```python
from build123d import *

# Parameters (mm, degrees)
BOSS_EXTRUDE1_DEPTH             = 3.175
F_6_CLEARANCE_HOLE1_AT_2_COUNT  = 2
F_6_CLEARANCE_HOLE1_AT_2_PITCH  = 202.184
F_6_CLEARANCE_HOLE1_AT_3_COUNT  = 2
F_6_CLEARANCE_HOLE1_AT_3_PITCH  = 245.533205315
F_6_CLEARANCE_HOLE1_AT_4_COUNT  = 2
F_6_CLEARANCE_HOLE1_AT_4_PITCH  = 294.732330958
F_6_CLEARANCE_HOLE1_AT_5_COUNT  = 2
F_6_CLEARANCE_HOLE1_AT_5_PITCH  = 209.296
F_6_CLEARANCE_HOLE1_AT_6_COUNT  = 2
F_6_CLEARANCE_HOLE1_AT_6_PITCH  = 172.811757411
F_6_CLEARANCE_HOLE1_AT_7_COUNT  = 2
F_6_CLEARANCE_HOLE1_AT_7_PITCH  = 57.300187604
F_6_CLEARANCE_HOLE1_AT_8_COUNT  = 2
F_6_CLEARANCE_HOLE1_AT_8_PITCH  = 291.003755082
F_6_CLEARANCE_HOLE1_AT_9_COUNT  = 2
F_6_CLEARANCE_HOLE1_AT_9_PITCH  = 232.431512666
F_6_CLEARANCE_HOLE1_AT_10_COUNT = 2
F_6_CLEARANCE_HOLE1_AT_10_PITCH = 101.092
SKETCH23_R                      = 24.765
CUT_EXTRUDE10_DEPTH             = 191.76187976
SKETCH24_W                      = 59.69
SKETCH24_H                      = 45.212
CUT_EXTRUDE11_DEPTH             = 191.76187976
FILLET2_R                       = 4.699
CHAMFER1_SIZE                   = 1.905
M3_CLEARANCE_HOLE3_AT_2_COUNT   = 2
M3_CLEARANCE_HOLE3_AT_2_PITCH   = 49.391408666
M3_CLEARANCE_HOLE3_AT_3_COUNT   = 2
M3_CLEARANCE_HOLE3_AT_3_PITCH   = 69.85
M3_CLEARANCE_HOLE3_AT_4_COUNT   = 2
M3_CLEARANCE_HOLE3_AT_4_PITCH   = 49.391408666
M3_CLEARANCE_HOLE1_D            = 3.6
M3_CLEARANCE_HOLE1_CSINK_D      = 5.7
M3_CLEARANCE_HOLE1_CSINK_ANGLE  = 90
M3_CLEARANCE_HOLE2_AT_2_COUNT   = 2
M3_CLEARANCE_HOLE2_AT_2_PITCH   = 56.70042
M3_CLEARANCE_HOLE2_AT_3_COUNT   = 2
M3_CLEARANCE_HOLE2_AT_3_PITCH   = 102.00589147
M3_CLEARANCE_HOLE2_AT_4_COUNT   = 2
M3_CLEARANCE_HOLE2_AT_4_PITCH   = 109.267844742
M3_CLEARANCE_HOLE2_AT_5_COUNT   = 2
M3_CLEARANCE_HOLE2_AT_5_PITCH   = 65.600653918
M3_CLEARANCE_HOLE2_AT_6_COUNT   = 2
M3_CLEARANCE_HOLE2_AT_6_PITCH   = 76.404880698
M3_CLEARANCE_HOLE2_AT_7_COUNT   = 2
M3_CLEARANCE_HOLE2_AT_7_PITCH   = 27.404059918
M3_CLEARANCE_HOLE2_AT_8_COUNT   = 2
M3_CLEARANCE_HOLE2_AT_8_PITCH   = 55.968061912
SKETCH35_W                      = 13.335
SKETCH35_H                      = 28.575
CUT_EXTRUDE12_DEPTH             = 191.76187976
FILLET1_R                       = 1.5875
F_8_0MM_DOWEL_HOLE1_D           = 8
M3_CLEARANCE_HOLE4_AT_2_COUNT   = 2
M3_CLEARANCE_HOLE4_AT_2_PITCH   = 78.105
M3_CLEARANCE_HOLE4_AT_3_COUNT   = 2
M3_CLEARANCE_HOLE4_AT_3_PITCH   = 97.157075141
M3_CLEARANCE_HOLE4_AT_4_COUNT   = 2
M3_CLEARANCE_HOLE4_AT_4_PITCH   = 57.785


with BuildPart() as part:
    # Sketch1 → Boss-Extrude1 (new body)
    with BuildSketch(Plane.XY):
        with BuildLine():
            Line((-151.96693, 98.7552), (-151.96693, -98.7552))
            ThreePointArc((-151.96693, -98.7552), (-147.131262957, -110.429532957), (-135.45693, -115.2652))
            Line((-135.45693, -115.2652), (135.45693, -115.2652))
            ThreePointArc((135.45693, -115.2652), (147.131262957, -110.429532957), (151.96693, -98.7552))
            Line((151.96693, -98.7552), (151.96693, 98.7552))
            ThreePointArc((151.96693, 98.7552), (147.131262957, 110.429532957), (135.45693, 115.2652))
            Line((135.45693, 115.2652), (-135.45693, 115.2652))
            ThreePointArc((-135.45693, 115.2652), (-147.131262957, 110.429532957), (-151.96693, 98.7552))
        make_face()
    extrude(amount=-BOSS_EXTRUDE1_DEPTH)

    # Sketch3 → #6 Clearance Hole1 (revolve, cut)
    with BuildSketch(Plane(origin=(101.092, 104.648, 0), x_dir=(0, -1, 0), z_dir=(1, 0, 0))):
        Polygon((0, 0), (0, 3.175), (3.3655, 3.175), (2.15265, 2.157298012), (2.15265, 0), align=None)
    f_6_clearance_hole1 = revolve(axis=Axis((101.092, 104.648, 6.35), (0, 0, -1)), mode=Mode.SUBTRACT)

    # #6 Clearance Hole1 at 2: #6 Clearance Hole1 ×2
    with Locations(*[(-i * F_6_CLEARANCE_HOLE1_AT_2_PITCH, 0, 0) for i in range(1, F_6_CLEARANCE_HOLE1_AT_2_COUNT)]):
        add(f_6_clearance_hole1, mode=Mode.SUBTRACT)

    # #6 Clearance Hole1 at 3: #6 Clearance Hole1 ×2
    with Locations(*[Vector(-0.9858574105677721, -0.1675862942743448, 0) * (i * F_6_CLEARANCE_HOLE1_AT_3_PITCH) for i in range(1, F_6_CLEARANCE_HOLE1_AT_3_COUNT)]):
        add(f_6_clearance_hole1, mode=Mode.SUBTRACT)

    # #6 Clearance Hole1 at 4: #6 Clearance Hole1 ×2
    with Locations(*[Vector(-0.8212900471859665, -0.5705108749123656, 0) * (i * F_6_CLEARANCE_HOLE1_AT_4_PITCH) for i in range(1, F_6_CLEARANCE_HOLE1_AT_4_COUNT)]):
        add(f_6_clearance_hole1, mode=Mode.SUBTRACT)

    # #6 Clearance Hole1 at 5: #6 Clearance Hole1 ×2
    with Locations(*[(0, -i * F_6_CLEARANCE_HOLE1_AT_5_PITCH, 0) for i in range(1, F_6_CLEARANCE_HOLE1_AT_5_COUNT)]):
        add(f_6_clearance_hole1, mode=Mode.SUBTRACT)

    # #6 Clearance Hole1 at 6: #6 Clearance Hole1 ×2
    with Locations(*[Vector(0.23075241289949347, -0.9730124993755537, 0) * (i * F_6_CLEARANCE_HOLE1_AT_6_PITCH) for i in range(1, F_6_CLEARANCE_HOLE1_AT_6_COUNT)]):
        add(f_6_clearance_hole1, mode=Mode.SUBTRACT)

    # #6 Clearance Hole1 at 7: #6 Clearance Hole1 ×2
    with Locations(*[Vector(0.6959266918172804, -0.7181128320927402, 0) * (i * F_6_CLEARANCE_HOLE1_AT_7_PITCH) for i in range(1, F_6_CLEARANCE_HOLE1_AT_7_COUNT)]):
        add(f_6_clearance_hole1, mode=Mode.SUBTRACT)

    # #6 Clearance Hole1 at 8: #6 Clearance Hole1 ×2
    with Locations(*[Vector(-0.6947814125038304, -0.719220959677332, 0) * (i * F_6_CLEARANCE_HOLE1_AT_8_PITCH) for i in range(1, F_6_CLEARANCE_HOLE1_AT_8_COUNT)]):
        add(f_6_clearance_hole1, mode=Mode.SUBTRACT)

    # #6 Clearance Hole1 at 9: #6 Clearance Hole1 ×2
    with Locations(*[Vector(-0.4349324187613887, -0.9004630981391565, 0) * (i * F_6_CLEARANCE_HOLE1_AT_9_PITCH) for i in range(1, F_6_CLEARANCE_HOLE1_AT_9_COUNT)]):
        add(f_6_clearance_hole1, mode=Mode.SUBTRACT)

    # #6 Clearance Hole1 at 10: #6 Clearance Hole1 ×2
    with Locations(*[(-i * F_6_CLEARANCE_HOLE1_AT_10_PITCH, 0, 0) for i in range(1, F_6_CLEARANCE_HOLE1_AT_10_COUNT)]):
        add(f_6_clearance_hole1, mode=Mode.SUBTRACT)

    # Sketch23 → Cut-Extrude10 (cut, through all)
    with BuildSketch(Plane.XY):
        with Locations((104.26573, 42.164)):
            Circle(SKETCH23_R)
    extrude(amount=-CUT_EXTRUDE10_DEPTH, mode=Mode.SUBTRACT)

    # Sketch24 → Cut-Extrude11 (cut, through all)
    with BuildSketch(Plane.XY):
        with Locations((-63.06693, 16.31442)):
            Rectangle(SKETCH24_W, SKETCH24_H)
    extrude(amount=-CUT_EXTRUDE11_DEPTH, mode=Mode.SUBTRACT)

    # Fillet2
    fillet2_edges = [part.edges().sort_by_distance(p)[0] for p in [
        (-92.91193, -6.29158, -1.5875),
        (-92.91193, 38.92042, -1.5875),
        (-33.22193, 38.92042, -1.5875),
        (-33.22193, -6.29158, -1.5875),
    ]]
    fillet(fillet2_edges, radius=FILLET2_R)

    # Chamfer1
    chamfer1_edges = [part.edges().sort_by_distance(p)[0] for p in [
        (-33.22193, 16.31442, -3.175),
        (-63.06693, -6.29158, -3.175),
        (-92.91193, 16.31442, -3.175),
        (-63.06693, 38.92042, -3.175),
        (-34.598235235, -4.915274765, -3.175),
        (-91.535624765, -4.915274765, -3.175),
        (-91.535624765, 37.544114765, -3.175),
        (-34.598235235, 37.544114765, -3.175),
    ]]
    chamfer(chamfer1_edges, length=CHAMFER1_SIZE)

    # Sketch30 → M3 Clearance Hole3 (revolve, cut)
    with BuildSketch(Plane(origin=(79.570025667, 66.859704333, 0), x_dir=(0, -1, 0), z_dir=(1, 0, 0))):
        Polygon((0, 0), (0, 3.175), (2.85, 3.175), (1.8, 2.125), (1.8, 0), align=None)
    m3_clearance_hole3 = revolve(axis=Axis((79.570025667, 66.859704333, 6.35), (0, 0, -1)), mode=Mode.SUBTRACT)

    # M3 Clearance Hole3 at 2: M3 Clearance Hole3 ×2
    with Locations(*[(i * M3_CLEARANCE_HOLE3_AT_2_PITCH, 0, 0) for i in range(1, M3_CLEARANCE_HOLE3_AT_2_COUNT)]):
        add(m3_clearance_hole3, mode=Mode.SUBTRACT)

    # M3 Clearance Hole3 at 3: M3 Clearance Hole3 ×2
    with Locations(*[Vector(0.7071067811865477, -0.7071067811865475, 0) * (i * M3_CLEARANCE_HOLE3_AT_3_PITCH) for i in range(1, M3_CLEARANCE_HOLE3_AT_3_COUNT)]):
        add(m3_clearance_hole3, mode=Mode.SUBTRACT)

    # M3 Clearance Hole3 at 4: M3 Clearance Hole3 ×2
    with Locations(*[(0, -i * M3_CLEARANCE_HOLE3_AT_4_PITCH, 0) for i in range(1, M3_CLEARANCE_HOLE3_AT_4_COUNT)]):
        add(m3_clearance_hole3, mode=Mode.SUBTRACT)

    # M3 Clearance Hole1 (through all)
    with Locations(Plane(origin=(0, 0, -3.175), x_dir=(-1, 0, 0), z_dir=(0, 0, -1))):
        with Locations((17.67693, -38.5952), (117.67693, -38.5952), (117.67693, -88.5952), (17.67693, -88.5952)):
            CounterSinkHole(M3_CLEARANCE_HOLE1_D / 2, M3_CLEARANCE_HOLE1_CSINK_D / 2, counter_sink_angle=M3_CLEARANCE_HOLE1_CSINK_ANGLE)

    # Sketch34 → M3 Clearance Hole2 (revolve, cut)
    with BuildSketch(Plane(origin=(25.25193, -75.5297, 0), x_dir=(0, -1, 0), z_dir=(1, 0, 0))):
        Polygon((0, 0), (0, 3.175), (2.85, 3.175), (1.8, 2.125), (1.8, 0), align=None)
    m3_clearance_hole2 = revolve(axis=Axis((25.25193, -75.5297, 6.35), (0, 0, -1)), mode=Mode.SUBTRACT)

    # M3 Clearance Hole2 at 2: M3 Clearance Hole2 ×2
    with Locations(*[(i * M3_CLEARANCE_HOLE2_AT_2_PITCH, 0, 0) for i in range(1, M3_CLEARANCE_HOLE2_AT_2_COUNT)]):
        add(m3_clearance_hole2, mode=Mode.SUBTRACT)

    # M3 Clearance Hole2 at 3: M3 Clearance Hole2 ×2
    with Locations(*[Vector(0.9983315525499471, -0.05774176290357108, 0) * (i * M3_CLEARANCE_HOLE2_AT_3_PITCH) for i in range(1, M3_CLEARANCE_HOLE2_AT_3_COUNT)]):
        add(m3_clearance_hole2, mode=Mode.SUBTRACT)

    # M3 Clearance Hole2 at 4: M3 Clearance Hole2 ×2
    with Locations(*[Vector(0.9319823250907686, 0.36250371821321364, 0) * (i * M3_CLEARANCE_HOLE2_AT_4_PITCH) for i in range(1, M3_CLEARANCE_HOLE2_AT_4_COUNT)]):
        add(m3_clearance_hole2, mode=Mode.SUBTRACT)

    # M3 Clearance Hole2 at 5: M3 Clearance Hole2 ×2
    with Locations(*[Vector(0.9959611085814934, -0.089785690358334, 0) * (i * M3_CLEARANCE_HOLE2_AT_5_PITCH) for i in range(1, M3_CLEARANCE_HOLE2_AT_5_COUNT)]):
        add(m3_clearance_hole2, mode=Mode.SUBTRACT)

    # M3 Clearance Hole2 at 6: M3 Clearance Hole2 ×2
    with Locations(*[Vector(0.8551246910281444, 0.5184223787550272, 0) * (i * M3_CLEARANCE_HOLE2_AT_6_PITCH) for i in range(1, M3_CLEARANCE_HOLE2_AT_6_COUNT)]):
        add(m3_clearance_hole2, mode=Mode.SUBTRACT)

    # M3 Clearance Hole2 at 7: M3 Clearance Hole2 ×2
    with Locations(*[Vector(0.2682084341495708, 0.9633609063331537, 0) * (i * M3_CLEARANCE_HOLE2_AT_7_PITCH) for i in range(1, M3_CLEARANCE_HOLE2_AT_7_COUNT)]):
        add(m3_clearance_hole2, mode=Mode.SUBTRACT)

    # M3 Clearance Hole2 at 8: M3 Clearance Hole2 ×2
    with Locations(*[Vector(0.8817603882311722, 0.47169759141468215, 0) * (i * M3_CLEARANCE_HOLE2_AT_8_PITCH) for i in range(1, M3_CLEARANCE_HOLE2_AT_8_COUNT)]):
        add(m3_clearance_hole2, mode=Mode.SUBTRACT)

    # Sketch35 → Cut-Extrude12 (cut, through all)
    with BuildSketch(Plane.XY):
        with Locations((-125.93193, 79.5782)):
            Rectangle(SKETCH35_W, SKETCH35_H)
    extrude(amount=-CUT_EXTRUDE12_DEPTH, mode=Mode.SUBTRACT)

    # Fillet1
    fillet1_edges = [part.edges().sort_by_distance(p)[0] for p in [
        (-132.59943, 65.2907, -1.5875),
        (-132.59943, 93.8657, -1.5875),
        (-119.26443, 93.8657, -1.5875),
        (-119.26443, 65.2907, -1.5875),
    ]]
    fillet(fillet1_edges, radius=FILLET1_R)

    # Ø8.0mm Dowel Hole1 (through all)
    with Locations(Plane(origin=(0, 0, -3.175), x_dir=(-1, 0, 0), z_dir=(0, 0, -1))):
        with Locations((12.26693, 3.61442), (12.26693, 29.01442)):
            Hole(F_8_0MM_DOWEL_HOLE1_D / 2)

    # Sketch39 → M3 Clearance Hole4 (revolve, cut)
    with BuildSketch(Plane(origin=(-105.23093, 45.65142, 0), x_dir=(0, -1, 0), z_dir=(1, 0, 0))):
        Polygon((0, 0), (0, 3.175), (2.85, 3.175), (1.7, 2.025), (1.7, 0), align=None)
    m3_clearance_hole4 = revolve(axis=Axis((-105.23093, 45.65142, 6.35), (0, 0, -1)), mode=Mode.SUBTRACT)

    # M3 Clearance Hole4 at 2: M3 Clearance Hole4 ×2
    with Locations(*[(i * M3_CLEARANCE_HOLE4_AT_2_PITCH, 0, 0) for i in range(1, M3_CLEARANCE_HOLE4_AT_2_COUNT)]):
        add(m3_clearance_hole4, mode=Mode.SUBTRACT)

    # M3 Clearance Hole4 at 3: M3 Clearance Hole4 ×2
    with Locations(*[Vector(0.8039043979705941, -0.5947585383359678, 0) * (i * M3_CLEARANCE_HOLE4_AT_3_PITCH) for i in range(1, M3_CLEARANCE_HOLE4_AT_3_COUNT)]):
        add(m3_clearance_hole4, mode=Mode.SUBTRACT)

    # M3 Clearance Hole4 at 4: M3 Clearance Hole4 ×2
    with Locations(*[(0, -i * M3_CLEARANCE_HOLE4_AT_4_PITCH, 0) for i in range(1, M3_CLEARANCE_HOLE4_AT_4_COUNT)]):
        add(m3_clearance_hole4, mode=Mode.SUBTRACT)


solid = part.part
```
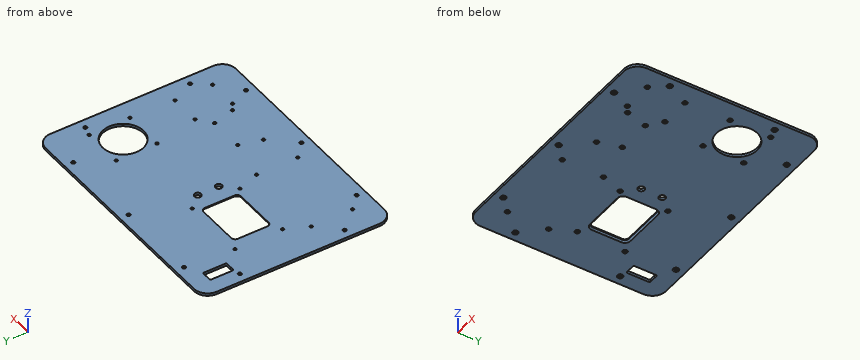
CAD build for the part. Positions are in the model's coordinates, mm. Round coordinates to 2 decimals unless told otherwise and drop trailing zeros. Write each loop counter-clockwise with the first axis right and the second up, starting at its lowest first coordinate (ties: lowest second). Pieces come first, ordered by that corner, then holes. Notation, with made-up numbers: (53.5, -36) -> (97.5, -36) arc R21 cw to (97.5, -22) -> close; hole circle Ø10 at (66.5, 4.5). An arc over 180 degrees is marked (long way). Answer in a Markdown table with one row per item. Add a question column.
Item 1: Drill centre lines: line 1 (Y direction, x = -1, z = -1.6); line 2 (X direction, y = -49, z = -0.6); line 3 (Y direction, x = -28.5, z = -0.8). Where is each one in solid material? Low to high. Write a range as from..to.
Item 2: Saw through at B-B, the plane y = 77.5. Write the cut outline in (x, z) (3 decimals), then the cut area to 3 significant figures.
Item 3: Drop flat-ended pins along their axis: pin 1 Ø6 at (x, y) = (79.57, 66.86) entering from +Z; pin 2 Ø7 at (x, y) = (-12.27, 29.01) entering from +Z. Give the stop position or say it passes through.
Item 4: Saw through at A-A, the plane x = -69. Write the cut outline in (y, z) (3 decimals), then the cut area to 3 significant figures.
Findings below:
| question | item | result |
|---|---|---|
| 1 | line 1 | y = -115.27..-106.55, -102.74..102.74, 106.55..115.27 |
| 1 | line 2 | x = -151.97..30.81, 34.4..72.81, 76.4..151.97 |
| 1 | line 3 | y = -115.27..-13.13, -11.13..44.65, 46.65..115.27 |
| 2 | outline | (-151.967, -3.175) -> (-132.599, -3.175) -> (-132.599, 0) -> (-151.967, 0) -> close; (-119.264, -3.175) -> (151.967, -3.175) -> (151.967, 0) -> (-119.264, 0) -> close |
| 2 | area | 923 mm^2 |
| 3 | pin 1 | stops at z = 0 |
| 3 | pin 2 | passes through |
| 4 | outline | (-115.265, -3.175) -> (-8.197, -3.175) -> (-6.292, -1.27) -> (-6.292, 0) -> (-115.265, 0) -> close; (38.92, -1.27) -> (40.825, -3.175) -> (115.265, -3.175) -> (115.265, 0) -> (38.92, 0) -> close |
| 4 | area | 585 mm^2 |
